from build123d import *

# Parameters (mm, degrees)
F0_R         = 3.5
F1_DEPTH     = 150
F3_DEPTH     = 5
F5_DEPTH     = 5
F6_R         = 5
F7_DEPTH     = 3
F8_F1_R      = 1
F8_F2_R      = 1
F8_T3_DEPTH  = 8
F8_T6_ANGLE  = 74.8218835265
F8_T7_DEPTH  = 8
F8_T10_ANGLE = 74.8218835265
F8_T11_DEPTH = 8
F8_T14_ANGLE = 74.8218835265
F8_T15_DEPTH = 8
F8_T18_ANGLE = 74.8218835265


# Not quite as in the source:
# - a fillet or chamfer that OpenCascade refuses, or shapes differently, is made with other operations: its cross-section is extruded or revolved along the edge and cut away or added


with BuildPart() as f1:
    # F0 (on Top) → F1 (new body)
    with BuildSketch(Plane.XY):
        Circle(F0_R)
    extrude(amount=F1_DEPTH)

    # F2 (on face) → F3 (join)
    with BuildSketch(Plane.XY.offset(150)):
        Polygon((5, -2.8867513459), (5, 2.8867513459), (0, 5.7735026919), (-5, 2.8867513459), (-5, -2.8867513459), (0, -5.7735026919), align=None)
    extrude(amount=F3_DEPTH)

    # F4 (on face) → F5 (join)
    with BuildSketch(Plane.XY.offset(155)):
        Polygon((6.5, -3.7527767497), (6.5, 3.7527767497), (0, 7.5055534995), (-6.5, 3.7527767497), (-6.5, -3.7527767497), (0, -7.5055534995), align=None)
    extrude(amount=F5_DEPTH)

    # F6 (on Right) → F7 (join, symmetric)
    with BuildSketch(Plane.YZ):
        with BuildLine():
            ThreePointArc((6, 168), (6.4085678246, 170.709769965), (7.5979446603, 173.1786084922))
            ThreePointArc((7.5979446603, 173.1786084922), (0, 183.6828522781), (-7.5979446603, 173.1786084922))
            ThreePointArc((-7.5979446603, 173.1786084922), (-6.4085678246, 170.709769965), (-6, 168))
            Line((-6, 168), (-6, 160))
            Line((-6, 160), (0, 160))
            Line((0, 160), (6, 160))
            Line((6, 160), (6, 168))
        make_face()
        with Locations((0, 175.6828522781)):
            Circle(F6_R, mode=Mode.SUBTRACT)
    extrude(amount=F7_DEPTH, both=True)

    # F8: fillet of radius 1 on 10 edges, made by hand

    # F8_f1
    f8_f1_edges = [f1.edges().sort_by_distance(p)[0] for p in [
        (3, 0, 183.6828522781),
    ]]
    fillet(f8_f1_edges, radius=F8_F1_R)

    # F8_f2
    f8_f2_edges = [f1.edges().sort_by_distance(p)[0] for p in [
        (-3, 0, 183.6828522781),
    ]]
    fillet(f8_f2_edges, radius=F8_F2_R)

    # F8_s4 → F8_t3 (cut)
    with BuildSketch(Plane.XY.offset(160)):
        with BuildLine():
            ThreePointArc((3, 5), (2.7071067812, 5.7071067812), (2, 6))
            Line((2, 6), (2, 6.02))
            Line((2, 6.02), (3.02, 6.02))
            Line((3.02, 6.02), (3.02, 5))
            Line((3.02, 5), (3, 5))
        make_face()
    extrude(amount=F8_T3_DEPTH, mode=Mode.SUBTRACT)

    # F8_s5 → F8_t6 (revolve, cut)
    with BuildSketch(Plane.XY.offset(168)):
        with BuildLine():
            ThreePointArc((2, 6), (2.7071067812, 5.7071067812), (3, 5))
            Line((3, 5), (3.02, 5))
            Line((3.02, 5), (3.02, 6.02))
            Line((3.02, 6.02), (2, 6.02))
            Line((2, 6.02), (2, 6))
        make_face()
    revolve(axis=Axis((3, 15.190372415, 168), (-1, 0, 0)), revolution_arc=F8_T6_ANGLE, mode=Mode.SUBTRACT)

    # F8_s8 → F8_t7 (cut)
    with BuildSketch(Plane.XY.offset(160)):
        with BuildLine():
            ThreePointArc((-2, 6), (-2.7071067812, 5.7071067812), (-3, 5))
            Line((-3, 5), (-3.02, 5))
            Line((-3.02, 5), (-3.02, 6.02))
            Line((-3.02, 6.02), (-2, 6.02))
            Line((-2, 6.02), (-2, 6))
        make_face()
    extrude(amount=F8_T7_DEPTH, mode=Mode.SUBTRACT)

    # F8_s9 → F8_t10 (revolve, cut)
    with BuildSketch(Plane.XY.offset(168)):
        with BuildLine():
            ThreePointArc((-2, 6), (-2.7071067812, 5.7071067812), (-3, 5))
            Line((-3, 5), (-3.02, 5))
            Line((-3.02, 5), (-3.02, 6.02))
            Line((-3.02, 6.02), (-2, 6.02))
            Line((-2, 6.02), (-2, 6))
        make_face()
    revolve(axis=Axis((-3, 15.190372415, 168), (-1, 0, 0)), revolution_arc=F8_T10_ANGLE, mode=Mode.SUBTRACT)

    # F8_s12 → F8_t11 (cut)
    with BuildSketch(Plane.XY.offset(160)):
        with BuildLine():
            ThreePointArc((-2, -6), (-2.7071067812, -5.7071067812), (-3, -5))
            Line((-3, -5), (-3.02, -5))
            Line((-3.02, -5), (-3.02, -6.02))
            Line((-3.02, -6.02), (-2, -6.02))
            Line((-2, -6.02), (-2, -6))
        make_face()
    extrude(amount=F8_T11_DEPTH, mode=Mode.SUBTRACT)

    # F8_s13 → F8_t14 (revolve, cut)
    with BuildSketch(Plane(origin=(0, -56.6005519955, 15.3548182499), x_dir=(1, 0, 0), z_dir=(0, -0.9651165645, 0.2618205815))):
        with BuildLine():
            ThreePointArc((-2, 167.3528031133), (-2.7071067812, 167.6456963322), (-3, 168.3528031133))
            Line((-3, 168.3528031133), (-3.02, 168.3528031133))
            Line((-3.02, 168.3528031133), (-3.02, 167.3328031133))
            Line((-3.02, 167.3328031133), (-2, 167.3328031133))
            Line((-2, 167.3328031133), (-2, 167.3528031133))
        make_face()
    revolve(axis=Axis((-3, -15.190372415, 168), (-1, 0, 0)), revolution_arc=F8_T14_ANGLE, mode=Mode.SUBTRACT)

    # F8_s16 → F8_t15 (cut)
    with BuildSketch(Plane.XY.offset(160)):
        with BuildLine():
            ThreePointArc((2, -6), (2.7071067812, -5.7071067812), (3, -5))
            Line((3, -5), (3.02, -5))
            Line((3.02, -5), (3.02, -6.02))
            Line((3.02, -6.02), (2, -6.02))
            Line((2, -6.02), (2, -6))
        make_face()
    extrude(amount=F8_T15_DEPTH, mode=Mode.SUBTRACT)

    # F8_s17 → F8_t18 (revolve, cut)
    with BuildSketch(Plane(origin=(0, -56.6005519955, 15.3548182499), x_dir=(1, 0, 0), z_dir=(0, -0.9651165645, 0.2618205815))):
        with BuildLine():
            ThreePointArc((2, 167.3528031133), (2.7071067812, 167.6456963322), (3, 168.3528031133))
            Line((3, 168.3528031133), (3.02, 168.3528031133))
            Line((3.02, 168.3528031133), (3.02, 167.3328031133))
            Line((3.02, 167.3328031133), (2, 167.3328031133))
            Line((2, 167.3328031133), (2, 167.3528031133))
        make_face()
    revolve(axis=Axis((3, -15.190372415, 168), (-1, 0, 0)), revolution_arc=F8_T18_ANGLE, mode=Mode.SUBTRACT)


solid = f1.part
Geometry: final body of the model. Coordinates: model frame, mm. A direction names the side the tool comes from. Give positions to 0.01 mm unless a question says otherwise; leave off trailing zeros. Loops run counter-clockwise (first coordinate to the right, second up) from the corner with the lowest first, then second, coordinate; pieces in that order, holes last. Notation, with made-up numbers: M 72.25,89.25 L 78.25,89.25 A24 cw 78.25,109.25 Z; hole C -2,-23 d7. An arc over 180 degrees is marked long. Put each result on its own line as item: value.
1) Cut plane B-B, the plane z = 151.5. Return the cut outline in (x, y).
Computed values:
outline: M -5,-2.89 L 0,-5.77 L 5,-2.89 L 5,2.89 L 0,5.77 L -5,2.89 Z
2) Mould query, pull axis Z, two halves, no side actions, for faces 6 (the cylindrical face through (-0.04, -1.08, 170.8)), 7 (the flat face through (0, -4, 150)), 8 (the flat face through (-2.465, 4.35, 152.465)). Classes: released by +Z, released by -Z, zero draft, split by the parting line, or undercut.
Computed values:
face 6: undercut
face 7: released by -Z
face 8: zero draft
3) Reachability of faces 1 (the flat face through (-5, 0, 152)), 2 (the cylindrical face through (0.028, 6.397, 170.673)), 3 (the cylindrical face through (3.233, -1.341, 73.95)), 4 (the flat face through (2.535, 4.31, 152.465)), 5 (the flat face through (5, 0, 152)) from +Z, -Z, +X, -X, +Y, -Y: full face, straight path, thin tool, end or side. Return the list, or none.
Computed values:
face 1: -Z, -X, +Y, -Y
face 2: +X, -X, +Y
face 3: -Z
face 4: -Z, +X, +Y
face 5: -Z, +X, +Y, -Y
4) Cut plane A-A, the plane y = 0. Return the cut outline in (x, z).
Computed values:
outline: M -6.5,155 L -5,155 L -5,150 L -3.5,150 L -3.5,0 L 3.5,0 L 3.5,150 L 5,150 L 5,155 L 6.5,155 L 6.5,160 L 3,160 L 3,170.68 L -3,170.68 L -3,160 L -6.5,160 Z; M -3,180.68 L 3,180.68 L 3,182.68 A1 ccw 2,183.68 L -2,183.68 A1 ccw -3,182.68 Z
5) First-contact query: P1, Ø2, axis at y = 6, z = 106.5, coming from the +X side; P2, Ø2, axis at y = 0.5, z = 20, coming from the -X side; P3, Ø2.5, axis at y = 0, z = 152.5, coming from the +X side; P4, Ø3, axis at x = -0.5, z = 163, coming from the -Y side. Flat tips, straight axial feed; report the tip coordinate or a pass-through.
Computed values:
P1: passes through
P2: stops at x = -3.5
P3: stops at x = 5
P4: stops at y = -6
6) Material intervals for L1, parallel to Z at x = -0.7, y = 0; L2, parallel to X at y = -7, z = 176; L3, parallel to Z at x = 5.75, y = -1.5, sorted ascending. Write a range as from..to.
Computed values:
L1: z = 0..170.68, 180.68..183.68
L2: x = -3..3
L3: z = 155..160
